```python
from build123d import *

# Parameters (mm, degrees)
BOSS_EXTRUDE1_DEPTH = 5
SKETCH2_R           = 4
CUT_EXTRUDE1_DEPTH  = 1
SKETCH3_R           = 2.25
CUT_EXTRUDE2_DEPTH  = 16
FILLET1_R           = 2


with BuildPart() as part:
    # Sketch1 → Boss-Extrude1 (new body)
    with BuildSketch(Plane.XY):
        Polygon((0, 0), (0, 42), (15, 42), (50.355339059, 6.644660941), (39.748737342, -3.961940777), (15, 20.786796564), (15, 0), align=None)
    extrude(amount=BOSS_EXTRUDE1_DEPTH)

    # Sketch2 → Cut-Extrude1 (cut)
    with BuildSketch(Plane.XY.offset(5)):
        with Locations((7.5, 10)):
            Circle(SKETCH2_R)
        with Locations((7.5, 32)):
            Circle(SKETCH2_R)
        with Locations((37.980970389, 8.412427894)):
            Circle(SKETCH2_R)
        with Locations((25.253048327, 21.140349955)):
            Circle(SKETCH2_R)
    extrude(amount=-CUT_EXTRUDE1_DEPTH, mode=Mode.SUBTRACT)

    # Sketch3 → Cut-Extrude2 (cut)
    with BuildSketch(Plane.XY.offset(4)):
        with Locations((7.5, 32)):
            Circle(SKETCH3_R)
        with Locations((7.5, 10)):
            Circle(SKETCH3_R)
        with Locations((25.253048327, 21.140349955)):
            Circle(SKETCH3_R)
        with Locations((37.980970389, 8.412427894)):
            Circle(SKETCH3_R)
    extrude(amount=-CUT_EXTRUDE2_DEPTH, mode=Mode.SUBTRACT)

    # Fillet1
    fillet1_edges = [part.edges().sort_by_distance(p)[0] for p in [
        (0, 0, 2.5),
        (0, 42, 2.5),
        (15, 42, 2.5),
        (50.355339059, 6.644660941, 2.5),
        (39.748737342, -3.961940777, 2.5),
        (15, 20.786796564, 2.5),
        (15, 0, 2.5),
    ]]
    fillet(fillet1_edges, radius=FILLET1_R)


solid = part.part
```
Input: part model. Units: mm. Frame: model coordinates. A direction names the side the tool comes from. Round coordinates to 2 decimals unless told otherwise and drop trailing zeros. Loops run counter-clockwise (first coordinate to the right, second up) from the corner with the lowest first, then second, coordinate; pieces in that order, holes last.
1) Section query C-C on x = 39. Return the cut outline in (y, z), plus the area to 3 significant figures.
Ans:
outline: (-2.99, 0) - (6.41, 0) - (6.41, 4) - (4.54, 4) - (4.54, 5) - (-2.99, 5) - close; (10.42, 0) - (18, 0) - (18, 5) - (12.28, 5) - (12.28, 4) - (10.42, 4) - close
area: 81.2 mm2
2) Section query A-A on y = 32. Return the cut outline in (x, z).
Ans:
outline: (0, 0) - (5.25, 0) - (5.25, 4) - (3.5, 4) - (3.5, 5) - (0, 5) - close; (9.75, 0) - (25, 0) - (25, 5) - (11.5, 5) - (11.5, 4) - (9.75, 4) - close
3) Material intervals for line 1 (Y direction, x = 7.5, z = 1.45); line 2 (Y direction, x = 7.5, z = 4.4); line 3 (Y direction, x = 3, z = 2.75), sorted ascending.
Ans:
line 1: y = 0 to 7.75, 12.25 to 29.75, 34.25 to 42
line 2: y = 0 to 6, 14 to 28, 36 to 42
line 3: y = 0 to 42
4) Section query B-B on x = 7.5. Return the cut outline in (y, z), plus the area to 3 significant figures.
Ans:
outline: (0, 0) - (7.75, 0) - (7.75, 4) - (6, 4) - (6, 5) - (0, 5) - close; (12.25, 0) - (29.75, 0) - (29.75, 4) - (28, 4) - (28, 5) - (14, 5) - (14, 4) - (12.25, 4) - close; (34.25, 0) - (42, 0) - (42, 5) - (36, 5) - (36, 4) - (34.25, 4) - close
area: 158 mm2
5) Set-up query: faces 5 (the flat face through (0, 21, 2)), 6 (the flat face through (9, 8, 4)), 7 (the flat face through (8, 0, 2)), 8 (the cylindrical face through (14.4, 0.57, 2.54)), 9 (the flat face through (32, 25, 2)). Return all of +Z, -Z, +X, -X, +Y, -Y with unobstructed straight access to the full face (end or side cutting, diameter ignored); none if empty.
Ans:
face 5: +Z, -Z, -X, +Y, -Y
face 6: +Z
face 7: +Z, -Z, -X, -Y
face 8: +Z, -Z, -Y
face 9: +Z, -Z, +X, +Y
6) Pin query (flat end, axial travel): pin 1 (5 mm diameter, centred on x = 37.98, y = 8.41, fed in from +Z); pin 2 (2.5 mm diameter, centred on x = 25, y = 20.5, fed in from +Z); pin 3 (2 mm diameter, centred on x = 6, z = 1, fed in from -Y); pin 4 (2 mm diameter, centred on x = 15, z = 4, fed in from -Y). Return the tip coordinate at first contact, or that it passes through.
Ans:
pin 1: stops at z = 4
pin 2: passes through
pin 3: stops at y = 0
pin 4: stops at y = 0.27
7) Pull-direction query (Y, two-part tool) for faces 1 (the flat face through (45.11, 1.4, 2.46)), 2 (the flat face through (20, 20, 0)), 3 (the flat face through (40, 7, 4)), 4 (the flat face through (9, 30, 4)); classes: released by +Y, released by -Y, zero draft, split by the parting line, or undercut.
Ans:
face 1: released by -Y
face 2: zero draft
face 3: undercut
face 4: undercut
8) Section query D-D on y = 10. Return the cut outline in (x, z), plus the area to 3 significant figures.
Ans:
outline: (0, 0) - (5.25, 0) - (5.25, 4) - (3.5, 4) - (3.5, 5) - (0, 5) - close; (9.75, 0) - (15, 0) - (15, 5) - (11.5, 5) - (11.5, 4) - (9.75, 4) - close; (25.79, 0) - (36.39, 0) - (36.39, 4) - (34.31, 4) - (34.31, 5) - (25.79, 5) - close; (39.58, 0) - (47, 0) - (47, 5) - (41.65, 5) - (41.65, 4) - (39.58, 4) - close
area: 135 mm2
